```python
from build123d import *

# Parameters (mm, degrees)
SKETCH1_W           = 53
SKETCH1_H           = 23
BOSS_EXTRUDE1_DEPTH = 2
SKETCH3_W           = 53
SKETCH3_H           = 23
SKETCH3_W_2         = 49
SKETCH3_H_2         = 19
BOSS_EXTRUDE2_DEPTH = 19
SKETCH5_W           = 53
SKETCH5_H           = 23
BOSS_EXTRUDE3_DEPTH = 2
CUT_EXTRUDE1_REACH  = 25
CUT_EXTRUDE2_REACH  = 55
CUT_EXTRUDE3_REACH  = 55
SKETCH9_W           = 19
SKETCH9_H           = 19
SKETCH10_W          = 2
SKETCH10_H          = 20
CUT_EXTRUDE4_DEPTH  = 21.5
FILLET1_R           = 1


with BuildPart() as part:
    # Sketch1 → Boss-Extrude1 (new body)
    with BuildSketch(Plane(origin=(0, 0, 0), x_dir=(1, 0, 0), z_dir=(0, 1, 0))):
        with Locations((26.5, 11.5)):
            Rectangle(SKETCH1_W, SKETCH1_H)
        with BuildLine():
            ThreePointArc((14.167979799, 11.103372859), (12.853372859, 10.582020201), (12.332020201, 11.896627141))
            add(Edge.make_bspline(
                [(12.332020201, 11.896627141), (12.469480865, 12.214775093), (12.762832878, 12.862826424), (13.335933972, 14.00565416), (14.069559606, 15.249143301), (14.976946321, 16.440651864), (16.244519266, 17.664776994), (18.013213928, 18.520696074), (20.198395592, 18.347411342), (22.11067197, 17.353298864), (24.473450461, 15.381830316), (26.713246554, 12.781426707), (28.903370071, 10.24854759), (30.508326384, 8.567330823), (32.048368225, 7.290846303), (33.447040029, 6.607713215), (34.391956609, 6.552903154), (35.163585916, 6.806063587), (35.804481551, 7.206405018), (36.50793545, 7.876095679), (37.256247569, 8.85306811), (37.906431149, 9.951709918), (38.429850366, 10.994805159), (38.704188556, 11.600765219), (38.832020201, 11.896627141)],
                knots=[0, 0, 0, 0, 0.015625, 0.03125, 0.0625, 0.09375, 0.125, 0.1875, 0.25, 0.3125, 0.375, 0.5, 0.5625, 0.625, 0.6875, 0.75, 0.8125, 0.84375, 0.875, 0.90625, 0.9375, 0.96875, 0.984375, 1, 1, 1, 1], degree=3))
            ThreePointArc((38.832020201, 11.896627141), (40.146627141, 12.417979799), (40.667979799, 11.103372859))
            add(Edge.make_bspline(
                [(14.167979799, 11.103372859), (14.295811444, 11.399234781), (14.570149634, 12.005194841), (15.093568851, 13.048290082), (15.743752431, 14.14693189), (16.49206455, 15.123904321), (17.195518449, 15.793594982), (17.836414084, 16.193936413), (18.608043391, 16.447096846), (19.552959971, 16.392286785), (20.951631775, 15.709153697), (22.491673616, 14.432669177), (24.096629929, 12.75145241), (26.286753446, 10.218573293), (28.526549539, 7.618169684), (30.88932803, 5.646701136), (32.801604408, 4.652588658), (34.986786072, 4.479303926), (36.755480734, 5.335223006), (38.023053679, 6.559348136), (38.930440394, 7.750856699), (39.664066028, 8.99434584), (40.237167122, 10.137173576), (40.530519135, 10.785224907), (40.667979799, 11.103372859)],
                knots=[0, 0, 0, 0, 0.015625, 0.03125, 0.0625, 0.09375, 0.125, 0.15625, 0.1875, 0.25, 0.3125, 0.375, 0.4375, 0.5, 0.625, 0.6875, 0.75, 0.8125, 0.875, 0.90625, 0.9375, 0.96875, 0.984375, 1, 1, 1, 1], degree=3))
        make_face(mode=Mode.SUBTRACT)
    extrude(amount=BOSS_EXTRUDE1_DEPTH)

    # Sketch3 → Boss-Extrude2 (add)
    with BuildSketch(Plane(origin=(0, 2, 0), x_dir=(1, 0, 0), z_dir=(0, 1, 0))):
        with Locations((26.5, 11.5)):
            Rectangle(SKETCH3_W, SKETCH3_H)
        with Locations((26.5, 11.5)):
            Rectangle(SKETCH3_W_2, SKETCH3_H_2, mode=Mode.SUBTRACT)
    extrude(amount=BOSS_EXTRUDE2_DEPTH)

    # Sketch5 → Boss-Extrude3 (add)
    with BuildSketch(Plane(origin=(0, 21, 0), x_dir=(1, 0, 0), z_dir=(0, 1, 0))):
        with Locations((26.5, 11.5)):
            Rectangle(SKETCH5_W, SKETCH5_H)
    extrude(amount=BOSS_EXTRUDE3_DEPTH)

    # Sketch7 → Cut-Extrude1 (cut, up to next)
    with BuildSketch(Plane(origin=(0, 23, 0), x_dir=(1, 0, 0), z_dir=(0, 1, 0)), mode=Mode.PRIVATE) as cut_extrude1_sk1:
        with BuildLine():
            ThreePointArc((12.334246428, 11.098259542), (12.848259542, 12.415753572), (14.165753572, 11.901740458))
            add(Edge.make_bspline(
                [(14.165753572, 11.901740458), (14.319569541, 11.551122241), (14.647608492, 10.832183671), (15.265371347, 9.591848537), (16.019360121, 8.279562849), (16.869534053, 7.103102818), (17.654222781, 6.289831839), (18.34890312, 5.806641268), (18.938193167, 5.587801008), (19.463132193, 5.549931301), (20.195435511, 5.70020599), (21.280226269, 6.347578401), (22.712802701, 7.841295003), (24.17836504, 9.816346352), (26.159265484, 12.791351284), (28.18067633, 15.841945555), (30.383820425, 18.160165201), (32.247719208, 19.361531089), (34.538967294, 19.56728313), (36.355209033, 18.558624621), (37.689381474, 17.159152284), (38.675063468, 15.789280734), (39.49940357, 14.351448085), (40.159389491, 13.025812725), (40.503651701, 12.271246104), (40.665753572, 11.901740458)],
                knots=[0, 0, 0, 0, 0.015625, 0.03125, 0.0625, 0.09375, 0.125, 0.15625, 0.1875, 0.21875, 0.25, 0.3125, 0.375, 0.4375, 0.5, 0.625, 0.6875, 0.75, 0.8125, 0.875, 0.90625, 0.9375, 0.96875, 0.984375, 1, 1, 1, 1], degree=3))
            ThreePointArc((40.665753572, 11.901740458), (40.151740458, 10.584246428), (38.834246428, 11.098259542))
            add(Edge.make_bspline(
                [(12.334246428, 11.098259542), (12.496348299, 10.728753896), (12.840610509, 9.974187275), (13.50059643, 8.648551915), (14.324936532, 7.210719266), (15.310618526, 5.840847716), (16.644790967, 4.441375379), (18.461032706, 3.43271687), (20.752280792, 3.638468911), (22.616179575, 4.839834799), (24.81932367, 7.158054445), (26.840734516, 10.208648716), (28.82163496, 13.183653648), (30.287197299, 15.158704997), (31.719773731, 16.652421599), (32.804564489, 17.29979401), (33.536867807, 17.450068699), (34.061806833, 17.412198992), (34.65109688, 17.193358732), (35.345777219, 16.710168161), (36.130465947, 15.896897182), (36.980639879, 14.720437151), (37.734628653, 13.408151463), (38.352391508, 12.167816329), (38.680430459, 11.448877759), (38.834246428, 11.098259542)],
                knots=[0, 0, 0, 0, 0.015625, 0.03125, 0.0625, 0.09375, 0.125, 0.1875, 0.25, 0.3125, 0.375, 0.5, 0.5625, 0.625, 0.6875, 0.75, 0.78125, 0.8125, 0.84375, 0.875, 0.90625, 0.9375, 0.96875, 0.984375, 1, 1, 1, 1], degree=3))
        make_face()
    cut_extrude1_tool1 = extrude(cut_extrude1_sk1.sketch, amount=-CUT_EXTRUDE1_REACH, mode=Mode.PRIVATE) & part.part
    add(cut_extrude1_tool1.solids().sort_by_distance((26.5, 23, -11.500446))[0], mode=Mode.SUBTRACT)

    # Sketch8 → Cut-Extrude2 (cut, up to next)
    with BuildSketch(Plane.ZY, mode=Mode.PRIVATE) as cut_extrude2_sk1:
        Polygon((-4, 8), (-4, 15), (-5.4, 15), (-7.1, 15.5), (-8.5, 15.5), (-8.5, 7.5), (-7.1, 7.5), (-5.4, 8), align=None)
    cut_extrude2_tool1 = extrude(cut_extrude2_sk1.sketch, amount=-CUT_EXTRUDE2_REACH, mode=Mode.PRIVATE) & part.part
    add(cut_extrude2_tool1.solids().sort_by_distance((0, 11.5, -6.321432))[0], mode=Mode.SUBTRACT)

    # Sketch9 → Cut-Extrude3 (cut, up to next)
    with BuildSketch(Plane(origin=(53, 0, 0), x_dir=(0, 0, -1), z_dir=(1, 0, 0)), mode=Mode.PRIVATE) as cut_extrude3_sk1:
        with Locations((11.5, 11.5)):
            Rectangle(SKETCH9_W, SKETCH9_H)
    cut_extrude3_tool1 = extrude(cut_extrude3_sk1.sketch, amount=-CUT_EXTRUDE3_REACH, mode=Mode.PRIVATE) & part.part
    add(cut_extrude3_tool1.solids().sort_by_distance((53, 11.5, -11.5))[0], mode=Mode.SUBTRACT)

    # Sketch10 → Cut-Extrude4 (cut)
    with BuildSketch(Plane(origin=(0, 23, 0), x_dir=(1, 0, 0), z_dir=(0, 1, 0))):
        with Locations((49, 11.5)):
            Rectangle(SKETCH10_W, SKETCH10_H)
    extrude(amount=-CUT_EXTRUDE4_DEPTH, mode=Mode.SUBTRACT)

    # Fillet1
    fillet1_edges = [part.edges().sort_by_distance(p)[0] for p in [
        (26.5, 0, -23),
        (53, 0, -11.5),
        (26.5, 0, 0),
        (0, 23, -11.5),
        (26.5, 23, 0),
        (53, 23, -11.5),
        (26.5, 23, -23),
        (0, 0, -11.5),
        (0, 11.5, -23),
        (53, 11.5, -23),
        (53, 11.5, 0),
        (0, 11.5, 0),
    ]]
    fillet(fillet1_edges, radius=FILLET1_R)


solid = part.part
```
Could you check a few things on this model? Use its own coordinates, in mm. A direction names the side the tool comes from. Round coordinates to 2 decimals unless told otherwise and drop trailing zeros. Write each loop counter-clockwise with the first axis right and the second up, starting at its lowest first coordinate (ties: lowest second). Pieces come first, ordered by that corner, then holes.
(1) If I drill on probe 1 along Y at (x, z) = (42.5, -2.25); probe 2 along Z at (x, y) = (4, 19.75); probe 3 along X at (y, z) = (1.75, -4.25), over which ranges is the centre line in solid material (lowest first)?
Findings below:
probe 1: y = 0 to 2, 21 to 23
probe 2: z = -23 to -21, -2 to 0
probe 3: x = 0 to 48, 50 to 53
(2) Which directions (+Z, -Z, +X, -X, +Y, -Y) give clear straight access to the entire face, cutting with the end or side of a thin tool? Please do faces 1 (the face through (52, 11, -2)), 2 (the face through (49, 12, -21.5)), 3 (the face through (1, 11, -4)).
Findings below:
face 1: +X
face 2: +Y
face 3: +X, -X
(3) Suppose I cut it at B-B on z = -2.75. Write out the boundary of the cut face in (x, y), and give its area (3 significant figures).
Findings below:
outline: (0, 1) arc R1 ccw to (1, 0) - (52, 0) arc R1 ccw to (53, 1) - (53, 2) - (50, 2) - (50, 1.5) - (48, 1.5) - (48, 2) - (2, 2) - (2, 21) - (48, 21) - (48, 23) - (1, 23) arc R1 ccw to (0, 22) - close; (50, 21) - (53, 21) - (53, 22) arc R1 ccw to (52, 23) - (50, 23) - close
area: 244 mm2
(4) Suppose I cut it at C-C on y = 19.25. Write out the boundary of the cut face in (x, z).
Findings below:
outline: (0, -22) arc R1 ccw to (1, -23) - (52, -23) arc R1 ccw to (53, -22) - (53, -21) - (50, -21) - (50, -21.5) - (48, -21.5) - (48, -21) - (2, -21) - (2, -2) - (48, -2) - (48, -1.5) - (50, -1.5) - (50, -2) - (53, -2) - (53, -1) arc R1 ccw to (52, 0) - (1, 0) arc R1 ccw to (0, -1) - close
(5) Suppose I cut it at D-D on z = -13.5. State how many separate pieces and enclosed holes the cut face has, and give its area (3 significant figures).
Findings below:
separate pieces: 6
enclosed holes: 0
area: 225 mm2
(6) Suppose I cut it at A-A on x = 44. Write out the boundary of the cut face in (y, z).
Findings below:
outline: (0, -22) arc R1 ccw to (1, -23) - (22, -23) arc R1 ccw to (23, -22) - (23, -1) arc R1 ccw to (22, 0) - (1, 0) arc R1 ccw to (0, -1) - close; hole (2, -21) - (21, -21) - (21, -2) - (2, -2) - close
(7) Thinking about a two-plate mould opening in Y: for faces 4 (the face through (25, 2, -9)), 5 (the face through (26, 11, 0)), 6 (the face through (26, 0, -14)), which applies, +Y half, -Y half, draft (parallel to the pull), parting line (faces both ways), or undercut?
Findings below:
face 4: undercut
face 5: draft
face 6: -Y half
(8) For pin 1 (8 mm diameter, centred on y = 6.5, z = -12, fed in from +X); pin 2 (8 mm diameter, centred on y = 13.5, z = -2.5, fed in from +X); pin 3 (0.7 mm diameter, centred on x = 0.5, z = -5, fed in from -Y), each with a flat end and sliding along its axis, tell me the tip position at first contact or that it passes through.
Findings below:
pin 1: stops at x = 2
pin 2: stops at x = 53
pin 3: stops at y = 0.01
